For this review, take the finished solid that the model builds, in its own axes (mm). A direction names the side the tool comes from. Round coordinates to 2 decimals unless told otherwise and drop trailing zeros. Loops run counter-clockwise (first coordinate to the right, second up) from the corner with the lowest first, then second, coordinate; pieces in that order, holes last. Notation, with made-up numbers: (-11, -2.5) -> (-3, -2.5) arc R14 cw to (-3, 17.5) -> close; hole circle Ø6 at (-19, 5.25). An arc over 180 degrees is marked (long way). Write each question's results on one line, items separated by ' | '.
Autodesk Inventor part; units mm, degrees
ref_plane "YZ Plane" through (0, 0, 0) normal (1, 0, 0) x (0, 1, 0)
ref_plane "XZ Plane" through (0, 0, 0) normal (0, 1, 0) x (-1, 0, 0)
ref_plane "XY Plane" through (0, 0, 0) normal (0, 0, 1) x (1, 0, 0)
sketch "Sketch1" plane through (0, 0, 0) normal (0, 0, 1) x (1, 0, 0)
  line L0 (-3.0031, 5) -> (3.0031, 5)
  arc A0 (-3.597, 4.8023) -> (-3.6, -4.8) centre (0, 0) ccw
  line L1 (3.0031, -5) -> (-3.0031, -5)
  arc A1 (-3.597, 4.8023) -> (-3.597, -4.8023) centre (0, 0) ccw
  arc A2 (3.597, -4.8023) -> (3.597, 4.8023) centre (0, 0) ccw
  arc A3 (-3.0031, 5) -> (-3.597, 4.8023) centre (-3.0031, 4.0094) ccw
  arc A4 (3.597, 4.8023) -> (3.0031, 5) centre (3.0031, 4.0094) ccw
  arc A5 (3.0031, -5) -> (3.597, -4.8023) centre (3.0031, -4.0094) ccw
  arc A6 (-3.597, -4.8023) -> (-3.0031, -5) centre (-3.0031, -4.0094) ccw
  point P0 (0, 0)
  point P1 (3.3166, 5)
  point P2 (3.3166, -5)
  point P3 (-3.3166, -5)
  dimension "d0" = 0.9906
extrude "Extrusion1" add sketch "Sketch1" along normal mid plane 19.9898
fillet "Fillet1" radius 0.508 8 edges at (-3.3161, 4.9493, 9.9949) (-6, 0, 9.9949) (-3.3161, -4.9493, 9.9949) (0, -5, 9.9949) (3.3161, -4.9493, 9.9949) (6, 0, 9.9949) (3.3161, 4.9493, 9.9949) (0, 5, 9.9949)
sketch "Sketch2" plane through (0, 0, 9.9949) normal (0, 0, 1) x (1, 0, 0)
  arc A0 (-3, 4.5) -> (-3.3, 4.4) centre (-2.9981, 3.9944) ccw
  spline S0 degree 3 poles (-3.3, 4.4) (-3.4685, 4.2736) (-3.6287, 4.1385) (-3.7806, 3.9947) (-3.8945, 3.8869) (-4.0038, 3.7742) (-4.1084, 3.6566) (-4.1433, 3.6174) (-4.1767, 3.5788) (-4.2115, 3.5374) (-4.4897, 3.2063) (-4.726, 2.8465) (-4.9194, 2.4597) (-5.0886, 2.1212) (-5.2214, 1.7694) (-5.3178, 1.4041) (-5.3315, 1.3519) (-5.3449, 1.298) (-5.3568, 1.2467) (-5.4522, 0.837) (-5.5, 0.4207) (-5.5, 0) (-5.5, -0.3681) (-5.4635, -0.7323) (-5.3904, -1.0926) (-5.38, -1.144) (-5.3691, -1.1941) (-5.3568, -1.2467) (-5.2588, -1.6679) (-5.1127, -2.0729) (-4.9194, -2.4597) (-4.7502, -2.7981) (-4.5484, -3.1155) (-4.3139, -3.4117) (-4.2805, -3.4541) (-4.2453, -3.4972) (-4.2115, -3.5374) (-3.941, -3.8595) (-3.6373, -4.147) (-3.3, -4.4) knots 0 0 0 0 0.0625 0.0625 0.0625 0.109375 0.109375 0.109375 0.125 0.125 0.125 0.25 0.25 0.25 0.359375 0.359375 0.359375 0.375 0.375 0.375 0.5 0.5 0.5 0.609375 0.609375 0.609375 0.625 0.625 0.625 0.75 0.75 0.75 0.859375 0.859375 0.859375 0.875 0.875 0.875 1 1 1 1
  arc A1 (-3.3, -4.4) -> (-3, -4.5) centre (-2.9981, -3.9944) ccw
  line L0 (-3, -4.5) -> (3, -4.5)
  arc A2 (3, -4.5) -> (3.3, -4.4) centre (2.9981, -3.9944) ccw
  arc A3 (3.3, -4.4) -> (3.3, 4.4) centre (0, 0) ccw
  arc A4 (3.3, 4.4) -> (3, 4.5) centre (2.9981, 3.9944) ccw
  line L1 (3, 4.5) -> (-3, 4.5)
  circle A5 centre (-4.25, 0) radius 0.7
  circle A6 centre (4.25, 0) radius 0.7
  circle A7 centre (0, 0) radius 2
  circle A8 centre (0, -3.5) radius 0.5
  circle A9 centre (0, -3.5) radius 0.5
  circle A10 centre (-4.25, 0) radius 0.7
  circle A11 centre (4.25, 0) radius 0.7
  circle A12 centre (0, 0) radius 2
  line L2 (3, 4.5) -> (-3, 4.5)
  arc A13 (-3, 4.5) -> (-3.3, 4.4) centre (-2.9981, 3.9944) ccw
  spline S1 degree 3 poles (-3.3, 4.4) (-3.4685, 4.2736) (-3.6287, 4.1385) (-3.7806, 3.9947) (-3.8945, 3.8869) (-4.0038, 3.7742) (-4.1084, 3.6566) (-4.1433, 3.6174) (-4.1767, 3.5788) (-4.2115, 3.5374) (-4.4897, 3.2063) (-4.726, 2.8465) (-4.9194, 2.4597) (-5.0886, 2.1212) (-5.2214, 1.7694) (-5.3178, 1.4041) (-5.3315, 1.3519) (-5.3449, 1.298) (-5.3568, 1.2467) (-5.4522, 0.837) (-5.5, 0.4207) (-5.5, 0) (-5.5, -0.3681) (-5.4635, -0.7323) (-5.3904, -1.0926) (-5.38, -1.144) (-5.3691, -1.1941) (-5.3568, -1.2467) (-5.2588, -1.6679) (-5.1127, -2.0729) (-4.9194, -2.4597) (-4.7502, -2.7981) (-4.5484, -3.1155) (-4.3139, -3.4117) (-4.2805, -3.4541) (-4.2453, -3.4972) (-4.2115, -3.5374) (-3.941, -3.8595) (-3.6373, -4.147) (-3.3, -4.4) knots 0 0 0 0 0.0625 0.0625 0.0625 0.109375 0.109375 0.109375 0.125 0.125 0.125 0.25 0.25 0.25 0.359375 0.359375 0.359375 0.375 0.375 0.375 0.5 0.5 0.5 0.609375 0.609375 0.609375 0.625 0.625 0.625 0.75 0.75 0.75 0.859375 0.859375 0.859375 0.875 0.875 0.875 1 1 1 1
  arc A14 (-3.3, -4.4) -> (-3, -4.5) centre (-2.9981, -3.9944) ccw
  line L3 (-3, -4.5) -> (3, -4.5)
  arc A15 (3, -4.5) -> (3.3, -4.4) centre (2.9981, -3.9944) ccw
  arc A16 (3.3, -4.4) -> (3.3, 4.4) centre (0, 0) ccw
  arc A17 (3.3, 4.4) -> (3, 4.5) centre (2.9981, 3.9944) ccw
  line L4 (-3, 5) -> (3, 5)
  arc A18 (3.6, -4.8) -> (3.6, 4.8) centre (0, 0) ccw
  arc A19 (-3.6, 4.8) -> (-3.6, -4.8) centre (0, 0) ccw
  line L5 (3, -5) -> (-3, -5)
  arc A20 (-3, 5) -> (-3.6, 4.8) centre (-3, 4) ccw
extrude "Extrusion2" add sketch "Sketch2" along normal blind 0.508 contours A7
fillet "Fillet2" radius 0.254 1 edges at (-2, 0, 10.5029)
extrude "Extrusion3" cut sketch "Sketch2" against normal blind 2.9972 contours A5 | A6 | A8
sketch "Sketch3" plane through (0, 0, 10.5029) normal (0, 0, 1) x (1, 0, 0)
  circle A0 centre (0, 0) radius 1.746
  circle A1 centre (0, 0) radius 0.4953
  dimension "d9" = 0.9906
extrude "Extrusion4" add sketch "Sketch3" along normal blind 4.4958 contours A1
fillet "Fillet3" radius 0.4953 1 edges at (-0.4953, 0, 14.9987)
sketch "Sketch4" plane through (0, 0, -9.9949) normal (0, 0, -1) x (-1, 0, 0)
  arc A0 (-3.597, 4.8023) -> (-3.597, -4.8023) centre (0, 0) ccw
  circle A1 centre (0, 0) radius 2.5019
  dimension "d13" = 5.0038
extrude "Extrusion5" add sketch "Sketch4" along normal blind 1.1938
sketch "Sketch5" plane through (0, 0, -9.9949) normal (0, 0, -1) x (-1, 0, 0)
  arc A0 (-3, 5) -> (-3.6, 4.8) centre (-3, 4) ccw
  arc A1 (-3.6, 4.8) -> (-3.6, -4.8) centre (0, 0) ccw
  arc A2 (-3.6, -4.8) -> (-3, -5) centre (-3, -4) ccw
  line L0 (3, -5) -> (-3, -5)
  arc A3 (3, -5) -> (3.6, -4.8) centre (3, -4) ccw
  arc A4 (3.6, -4.8) -> (3.6, 4.8) centre (0, 0) ccw
  arc A5 (3.6, 4.8) -> (3, 5) centre (3, 4) ccw
  line L1 (-3, 5) -> (3, 5)
  line L2 (3.7, -1.0714) -> (3.7, 1.0714)
  line L3 (3.4, -1.0714) -> (3.7, -1.0714)
  line L4 (3.4, 1.0714) -> (3.4, -1.0714)
  line L5 (3.7, 1.0714) -> (3.4, 1.0714)
  circle A6 centre (0, 0) radius 2.5
  line L6 (-3.7, -1.0714) -> (-3.4, -1.0714)
  line L7 (-3.7, 1.0714) -> (-3.7, -1.0714)
  line L8 (-3.4, 1.0714) -> (-3.7, 1.0714)
  line L9 (-3.4, -1.0714) -> (-3.4, 1.0714)
extrude "Extrusion6" add sketch "Sketch5" along normal blind 1.6002 contours L3 L4 L5 L2 | L7 L8 L9 L6
chamfer "Chamfer1" distance 0.508 angle 45 4 edges at (3.55, 1.0714, -11.5951) (3.55, -1.0714, -11.5951) (-3.55, 1.0714, -11.5951) (-3.55, -1.0714, -11.5951)
properties part number "QFK-N30QAV-16068"
1. Tool access review of faces 4 (the face through (3.7, 0, -11)), 5 (the face through (4, 0, 6.998)), 6 (the face through (0, 0, -11.189)): name each direction out of +Z, -Z, +X, -X, +Y, -Y from which nothing blocks a thin tool from reaching the whole face with its end or side.
Values found:
face 4: -Z, +X, +Y, -Y | face 5: +Z | face 6: -Z, +Y, -Y
2. Draft analysis for pull direction Y (two halves, no side actions). For faces 1 (the face through (0, -3, 9)), 2 (the face through (0, -5, 0)), 3 (the face through (-3.4, 0, -11)), state which applies: released by +Y, released by -Y, zero draft, split by the parting line, or undercut.
Values found:
face 1: undercut | face 2: released by -Y | face 3: zero draft
3. For pin 1 (1.3 mm diameter, centred on y = 0, z = -11, fed in from -X); pin 2 (0.8 mm diameter, centred on x = -4.25, y = 0, fed in from +Z); pin 3 (4 mm diameter, centred on y = 1.5, z = -1, fed in from +X); pin 4 (3 mm diameter, centred on x = -4.5, y = 3.5, fed in from +Z), all flat-tipped, find the tip position at first contact; note any pin that passes through.
Values found:
pin 1: stops at x = -3.7 | pin 2: stops at z = 7 | pin 3: stops at x = 6 | pin 4: stops at z = 9.99
4. Consider section B-B (z = 12). State the section outline as (x, y) points, plus the area to 3 significant figures.
Values found:
outline: circle Ø0.99 at (0, 0) | area: 0.771 mm2
5. To check wall thickness, follow probe 1 along Y at (x, z) = (0, 8); probe 2 along Y at (x, z) = (4.25, 8.1); probe 3 along Z at (x, y) = (0.5, 2.5). State the ranges of each line that lie inside material, in increasing order.
Values found:
probe 1: y = -5 to -4, -3 to 5 | probe 2: y = -4.24 to -0.7, 0.7 to 4.24 | probe 3: z = -9.99 to 9.99
6. Consider section A-A (x = 0). State the section outline as (y, z) points.
Values found:
outline: (-5, -9.99) -> (-2.5, -9.99) -> (-2.5, -11.19) -> (2.5, -11.19) -> (2.5, -9.99) -> (5, -9.99) -> (5, 9.49) arc R0.51 ccw to (4.49, 9.99) -> (2, 9.99) -> (2, 10.25) arc R0.25 ccw to (1.75, 10.5) -> (0.5, 10.5) -> (0.5, 14.5) arc R0.5 ccw to (-0.5, 14.5) -> (-0.5, 10.5) -> (-1.75, 10.5) arc R0.25 ccw to (-2, 10.25) -> (-2, 9.99) -> (-3, 9.99) -> (-3, 7) -> (-4, 7) -> (-4, 9.99) -> (-4.49, 9.99) arc R0.51 ccw to (-5, 9.49) -> close
